Check sheet for the drawn part. Datum: minimum x, y, z corner. Units: mm. A direction names the side the tool comes from. Round coordinates to 2 decimals unless told otherwise and drop trailing zeros. Loops run counter-clockwise (first coordinate to the right, second up) from the corner with the lowest first, then second, coordinate; pieces in that order, holes last. Notation, with made-up numbers: (38.5, -6.75) -> (54.5, -6.75) arc R8 cw to (54.5, 0.25) -> close; hole circle Ø6 at (-13.5, -26). An arc over 180 degrees is marked (long way). Use CSV: the item, a comma, the result in double quotes. Start each with the question number.
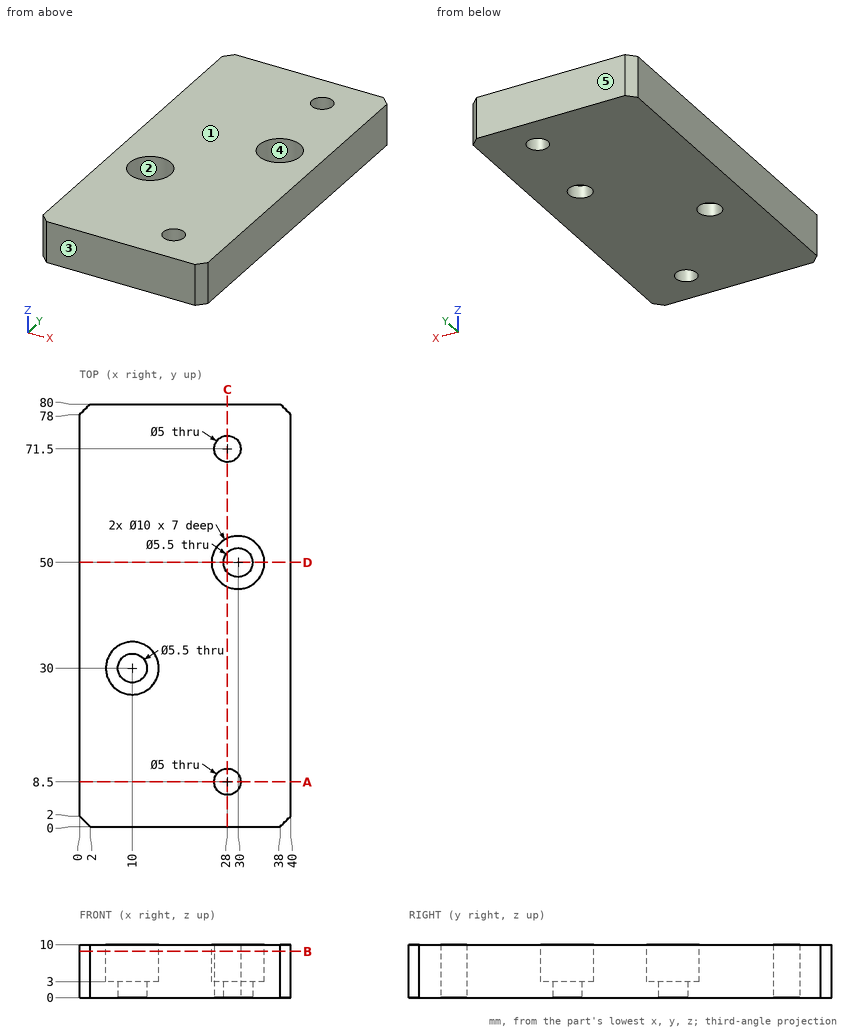
Q1. Cross-section at B-B (z = 8.75). Record the boundary of the cut face in (x, y).
Q2. Cross-section at A-A (y = 8.5). Record the boundary of the cut face in (x, z), and give its area (3 significant figures).
Q3. Cross-section at D-D (y = 50). Record the boundary of the cut face in (x, z), and give its area (4 significant figures).
Q4. Release check for a two-part mould opening along Y. For the marked faces 3, 4 and 5 record: +Y half, -Y half, draft (parallel to the pull), parting line (faces both ways), or undercut.
Q5. Depth check by flat-ended pin: pin 1 Ø3 at (x, y) = (32.5, 48.5) entering from -Z; pin 2 Ø5 at (x, y) = (31.5, 49) entering from +Z. Enter the tip coordinate at first touch or a pass-through.
Q6. Thickness scan on L1, parallel to Y at x = 28, z = 5.25; L2, parallel to Y at x = 30, z = 1.25; L3, parallel to Y at x = 10, z = 1.1. Record the ranges inside material, lowest first. Write a range as from..to.
Q7. Tool access check on the marked faces 1 and 2. Record the directions out of +Z, -Z, +X, -X, +Y, -Y that give a thin tool (end or side, any length) a straight path to the whole face; none if there is none.
Q8. Cross-section at C-C (x = 28). Record the boundary of the cut face in (y, z).
Answer list:
1,outline,"(0, 2) -> (2, 0) -> (38, 0) -> (40, 2) -> (40, 78) -> (38, 80) -> (2, 80) -> (0, 78) -> close; hole circle Ø10 at (10, 30); hole circle Ø10 at (30, 50); hole circle Ø5 at (28, 8.5); hole circle Ø5 at (28, 71.5)"
2,outline,"(0, 0) -> (25.5, 0) -> (25.5, 10) -> (0, 10) -> close; (30.5, 0) -> (40, 0) -> (40, 10) -> (30.5, 10) -> close"
2,area,"350 mm2"
3,outline,"(0, 0) -> (27.25, 0) -> (27.25, 3) -> (25, 3) -> (25, 10) -> (0, 10) -> close; (32.75, 0) -> (40, 0) -> (40, 10) -> (35, 10) -> (35, 3) -> (32.75, 3) -> close"
3,area,"313.5 mm2"
4,face 3,"-Y half"
4,face 4,"undercut"
4,face 5,"+Y half"
5,pin 1,"stops at z = 0"
5,pin 2,"stops at z = 3"
6,L1,"y = 0..6, 11..45.42, 54.58..69, 74..80"
6,L2,"y = 0..7, 10..47.25, 52.75..70, 73..80"
6,L3,"y = 0..27.25, 32.75..80"
7,face 1,"+Z, +X, -X, +Y, -Y"
7,face 2,"+Z"
8,outline,"(0, 0) -> (6, 0) -> (6, 10) -> (0, 10) -> close; (11, 0) -> (48.11, 0) -> (48.11, 3) -> (45.42, 3) -> (45.42, 10) -> (11, 10) -> close; (51.89, 0) -> (69, 0) -> (69, 10) -> (54.58, 10) -> (54.58, 3) -> (51.89, 3) -> close; (74, 0) -> (80, 0) -> (80, 10) -> (74, 10) -> close"
